Read the model definition and answer for the solid it produces. Units are mm, in the model's axes. A direction names the side the tool comes from. Coordinates: 2 decimals unless noted, no trailing zeros. Loops run counter-clockwise (first coordinate to the right, second up) from the corner with the lowest first, then second, coordinate; pieces in that order, holes last. Notation, with made-up numbers: M 65.5,82 L 75.5,82 A11 cw 75.5,88 Z; hole C 6.5,44 d10. An arc over 180 degrees is marked long. Use one line per item in the form item = value. Start each with the question number.
1. The part is cut by section D-D (z = 7.5). Give the vertices of the cut face in (x, y).
2. For a pull along X with two mould halves and no side action, classify faces 1 (the cylindrical face through (-63.427, -5.555, 42.487)), 2 (the flat face through (-58, -8.662, 23)) as released by +X, released by -X, zero draft, split by the parting line, or undercut.
3. The part is cut by section C-C (z = 41). Give the number of separate pieces and of enclosed holes in the cut face, plus the area to 3 significant figures.
4. Find the intervals of material crossed by probe 1 along X at (y, z) = (-1.75, 3.5); probe 2 along X at (y, z) = (-1.25, 27); probe 3 along Z at (x, y) = (-62.5, 1.75), in increasing order. Write a range as [from, to].
5. A tool of negligible diameter and unlimited length cuts with its end or side. For faces 3 (the cylindrical face through (-70.738, -3.957, 14.79)), 4 (the flat face through (-47.266, -7.676, 38.607)), 5 (the cylindrical face through (-53.771, -4.373, 42.877)), 6 (the flat face through (-58, 2, 0)), from which of +Z, -Z, +X, -X, +Y, -Y can it reach the whole face along a straight path? Write none if from no direction.
6. Flat-ended cylindrical pins translate along their axes: pin 1 (1.5 mm diameter, centred on y = 6, z = 43, fed in from -X); pin 2 (1.6 mm diameter, centred on y = -7.5, z = 40.5, fed in from +X); pin 3 (12 mm diameter, centred on y = 8, z = 31.5, fed in from +X). Find the tip coordinate at first contact, or state that the pin passes through.
7. The part is cut by section B-B (x = -58). Give the vertices of the cut face in (y, z), plus the area to 3 significant figures.
8. The part is cut by section A-A (z = 26). Give the vertices of the cut face in (x, y).
from build123d import *

# Parameters (mm, degrees)
SKETCH1_R           = 6.25
SKETCH1_R_2         = 4.15
BOSS_EXTRUDE1_DEPTH = 50
CUT_EXTRUDE1_DEPTH  = 127
BOSS_EXTRUDE2_DEPTH = 20
SKETCH4_R           = 6.25
CUT_EXTRUDE2_DEPTH  = 20
CUT_EXTRUDE3_START  = -30
SKETCH5_R           = 6.25
CUT_EXTRUDE3_DEPTH  = 30
FILLET1_R           = 3
SKETCH6_R           = 4.5
BOSS_EXTRUDE3_DEPTH = 30
SKETCH7_R           = 1.5
CUT_EXTRUDE4_DEPTH  = 30
CUT_EXTRUDE5_DEPTH  = 2
CUT_EXTRUDE6_START  = -30
SKETCH9_R           = 4.5
CUT_EXTRUDE6_DEPTH  = 30


with BuildPart() as part:
    # Sketch1 → Boss-Extrude1 (new body)
    with BuildSketch(Plane.XY):
        with BuildLine():
            Line((-73.62208004, 11.83829087), (106.37791996, 11.83829087))
            ThreePointArc((106.37791996, 11.83829087), (116.62791996, 1.58829087), (106.37791996, -8.66170913))
            Line((106.37791996, -8.66170913), (-73.62208004, -8.66170913))
            ThreePointArc((-73.62208004, -8.66170913), (-83.87208004, 1.58829087), (-73.62208004, 11.83829087))
        make_face()
        with Locations((-73.62208004, 1.58829087)):
            Circle(SKETCH1_R, mode=Mode.SUBTRACT)
        with Locations((-43.62208004, 1.58829087)):
            Circle(SKETCH1_R_2, mode=Mode.SUBTRACT)
        with Locations(Location((76.37791996, 1.58829087, 0), (0, 0, 180))):
            Circle(SKETCH1_R_2, mode=Mode.SUBTRACT)
        with Locations(Location((106.37791996, 1.58829087, 0), (0, 0, 180))):
            Circle(SKETCH1_R, mode=Mode.SUBTRACT)
    extrude(amount=BOSS_EXTRUDE1_DEPTH)

    # Sketch2 → Cut-Extrude1 (cut)
    with BuildSketch(Plane.XY.offset(50)):
        with BuildLine():
            Line((-43.62208004, 11.83829087), (132.206329773, 11.83829087))
            Line((132.206329773, 11.83829087), (132.206329773, -8.66170913))
            Line((132.206329773, -8.66170913), (-43.62208004, -8.66170913))
            ThreePointArc((-43.62208004, -8.66170913), (-33.37208004, 1.58829087), (-43.62208004, 11.83829087))
        make_face()
    extrude(amount=-CUT_EXTRUDE1_DEPTH, mode=Mode.SUBTRACT)

    # Sketch3 → Boss-Extrude2 (add)
    with BuildSketch(Plane.XY.offset(50)):
        with BuildLine():
            Line((-43.62208004, 11.83829087), (-73.62208004, 11.83829087))
            ThreePointArc((-73.62208004, 11.83829087), (-83.87208004, 1.58829087), (-73.62208004, -8.66170913))
            Line((-73.62208004, -8.66170913), (-43.62208004, -8.66170913))
            ThreePointArc((-43.62208004, -8.66170913), (-33.37208004, 1.58829087), (-43.62208004, 11.83829087))
        make_face()
    extrude(amount=-BOSS_EXTRUDE2_DEPTH)

    # Sketch4 → Cut-Extrude2 (cut)
    with BuildSketch(Plane.ZY.offset(43.62208004)):
        with Locations(Location((41, 1.58829087, 0), (0, 0, 270))):
            Circle(SKETCH4_R)
    extrude(amount=-CUT_EXTRUDE2_DEPTH, mode=Mode.SUBTRACT)

    # Sketch5 → Cut-Extrude3 (cut)
    with BuildSketch(Plane(origin=(-43.62208004, 0, 0), x_dir=(0, 0, -1), z_dir=(1, 0, 0)).offset(CUT_EXTRUDE3_START)):
        with Locations(Location((-41, 1.58829087, 0), (0, 0, 270))):
            Circle(SKETCH5_R)
    extrude(amount=CUT_EXTRUDE3_DEPTH, mode=Mode.SUBTRACT)

    # Fillet1
    # the kernel refuses this fillet: 3 mm, written as the material it takes off along each edge
    with BuildSketch(Plane(origin=(-73.62208004, 11.83829087, 50), x_dir=(0, 0, -1), z_dir=(1, 0, 0)), Plane(origin=(-43.62208004, -8.66170913, 50), x_dir=(0, 0, -1), z_dir=(-1, 0, 0))) as fillet1_piece_1:
        with BuildLine():
            CenterArc((FILLET1_R, -FILLET1_R), FILLET1_R, 90, 90)
            Line((0, -FILLET1_R), (0, 0))
            Line((0, 0), (FILLET1_R, 0))
        make_face()
    extrude(amount=30, mode=Mode.SUBTRACT)
    with BuildSketch(Plane(origin=(-73.62208004, 1.58829087, 50), x_dir=(0, -1, 0), z_dir=(1, 0, 0))) as fillet1_piece_2:
        with BuildLine():
            CenterArc((10.25 - FILLET1_R, FILLET1_R), FILLET1_R, 270, 90)
            Line((10.25, FILLET1_R), (10.25, 0))
            Line((10.25, 0), (10.25 - FILLET1_R, 0))
        make_face()
    revolve(axis=Axis((-73.62208004, 1.58829087, 50), (0, 0, -1)), revolution_arc=180, mode=Mode.SUBTRACT)
    with BuildSketch(Plane(origin=(-43.62208004, 1.58829087, 50), x_dir=(0, -1, 0), z_dir=(-1, 0, 0))) as fillet1_piece_3:
        with BuildLine():
            CenterArc((10.25 - FILLET1_R, -FILLET1_R), FILLET1_R, 0, 90)
            Line((10.25 - FILLET1_R, 0), (10.25, 0))
            Line((10.25, 0), (10.25, -FILLET1_R))
        make_face()
    revolve(axis=Axis((-43.62208004, 1.58829087, 50), (0, 0, 1)), revolution_arc=180, mode=Mode.SUBTRACT)

    # Sketch6 → Boss-Extrude3 (add)
    with BuildSketch(Plane(origin=(0, 0, 30), x_dir=(-1, 0, 0), z_dir=(0, 0, -1))):
        with Locations(Location((73.62208004, 1.58829087, 0), (0, 0, 180))):
            Circle(SKETCH6_R)
    extrude(amount=BOSS_EXTRUDE3_DEPTH)

    # Sketch7 → Cut-Extrude4 (cut)
    with BuildSketch(Plane(origin=(0, 11.83829087, 0), x_dir=(1, 0, 0), z_dir=(0, 1, 0))):
        with Locations(Location((-48.62208004, -41, 0), (0, 0, 180))):
            Circle(SKETCH7_R)
        with Locations(Location((-63.62208004, -41, 0), (0, 0, 180))):
            Circle(SKETCH7_R)
        with Locations(Location((-73.62208004, -26, 0), (0, 0, 180))):
            Circle(SKETCH7_R)
        with Locations(Location((-73.62208004, -5, 0), (0, 0, 180))):
            Circle(SKETCH7_R)
    extrude(amount=-CUT_EXTRUDE4_DEPTH, mode=Mode.SUBTRACT)

    # Sketch8 → Cut-Extrude5 (cut)
    with BuildSketch(Plane(origin=(0, -8.66170913, 0), x_dir=(-1, 0, 0), z_dir=(0, -1, 0))):
        Polygon((73.62208004, -8.175426481), (76.37208004, -6.58771324), (76.37208004, -3.41228676), (73.62208004, -1.824573519), (70.87208004, -3.41228676), (70.87208004, -6.58771324), align=None)
        Polygon((73.62208004, -29.175426481), (76.37208004, -27.58771324), (76.37208004, -24.41228676), (73.62208004, -22.824573519), (70.87208004, -24.41228676), (70.87208004, -27.58771324), align=None)
        Polygon((63.62208004, -44.175426481), (66.37208004, -42.58771324), (66.37208004, -39.41228676), (63.62208004, -37.824573519), (60.87208004, -39.41228676), (60.87208004, -42.58771324), align=None)
        Polygon((48.62208004, -44.175426481), (51.37208004, -42.58771324), (51.37208004, -39.41228676), (48.62208004, -37.824573519), (45.87208004, -39.41228676), (45.87208004, -42.58771324), align=None)
    extrude(amount=-CUT_EXTRUDE5_DEPTH, mode=Mode.SUBTRACT)

    # Sketch9 → Cut-Extrude6 (cut)
    with BuildSketch(Plane(origin=(0, 0, 0), x_dir=(-1, 0, 0), z_dir=(0, 0, -1)).offset(CUT_EXTRUDE6_START)):
        with Locations((73.62208004, 1.58829087)):
            Circle(SKETCH9_R)
    extrude(amount=CUT_EXTRUDE6_DEPTH, mode=Mode.SUBTRACT)


solid = part.part
Computed values:
q1.outline = M -74.79,-8.59 L -74.79,-6.66 L -72.45,-6.66 L -72.45,-8.66 L -43.62,-8.66 A10.25 ccw -43.62,11.84 L -73.62,11.84 A10.25 ccw Z; hole C -73.62,1.59 d12.5; hole C -43.62,1.59 d8.3
q2.face_1 = undercut
q2.face_2 = zero draft
q3.separate_pieces = 5
q3.enclosed_holes = 0
q3.area = 392 mm²
q4.probe_1 = [-83.31, -78.91], [-68.34, -46.09], [-41.16, -33.93]
q4.probe_2 = [-83.47, -79.19], [-68.05, -46.65], [-40.59, -33.77]
q4.probe_3 = [0, 34.75], [47.25, 50]
q5.face_3 = -Z
q5.face_4 = -Y
q5.face_5 = +X
q5.face_6 = -Z, +X, -X, +Y, -Y
q6.pin_1 = -83.2
q6.pin_2 = -37.59
q6.pin_3 = -33.38
q7.outline = M -8.66,0 L 11.84,0 L 11.84,47 A3 ccw 8.84,50 L -5.66,50 A3 ccw -8.66,47 Z; hole C 1.59,41 d12.5
q7.area = 898 mm²
q8.outline = M -76.37,-8.29 L -76.37,-6.66 L -75.12,-6.66 L -75.12,-4.48 A6.25 cw -75.12,7.66 L -75.12,11.73 A10.25 ccw Z; M -72.12,-6.66 L -70.87,-6.66 L -70.87,-8.66 L -43.62,-8.66 A10.25 ccw -43.62,11.84 L -72.12,11.84 L -72.12,7.66 A6.25 cw -72.12,-4.48 Z; hole C -43.62,1.59 d8.3
